from build123d import *

# Parameters (mm, degrees)
F0_R     = 3.175
F0_R_2   = 1.5875
F1_DEPTH = 25.4


with BuildPart() as f1:
    # F0 (on Front) → F1 (new body)
    with BuildSketch(Plane.XZ):
        with BuildLine():
            ThreePointArc((-9.525, 70.523976), (0, 60.998976), (9.525, 70.523976))
            ThreePointArc((9.525, 70.523976), (0, 80.048976), (-9.525, 70.523976))
        make_face()
        with Locations((0, 70.523976)):
            Circle(F0_R, mode=Mode.SUBTRACT)
        with BuildLine():
            Line((15.747457, 21.732266), (9.525, 70.523976))
            ThreePointArc((9.525, 70.523976), (0, 60.998976), (-9.525, 70.523976))
            Line((-9.525, 70.523976), (-15.747457, 21.732266))
            ThreePointArc((-15.747457, 21.732266), (0, 35.598976), (15.747457, 21.732266))
        make_face()
        with Locations((-4.959356, 56.249176)):
            Circle(F0_R_2, mode=Mode.SUBTRACT)
        with BuildLine():
            ThreePointArc((15.875, 19.723976), (15.843082, 20.730144), (15.747457, 21.732266))
            ThreePointArc((15.747457, 21.732266), (0, 35.598976), (-15.747457, 21.732266))
            ThreePointArc((-15.747457, 21.732266), (-15.873668, 19.929643), (-15.794203, 18.124357))
            ThreePointArc((-15.794203, 18.124357), (0, 3.848976), (15.794203, 18.124357))
            ThreePointArc((15.794203, 18.124357), (15.854788, 18.923147), (15.875, 19.723976))
        make_face()
        with Locations((0, 19.723976)):
            Circle(F0_R, mode=Mode.SUBTRACT)
        with BuildLine():
            ThreePointArc((15.794203, 18.124357), (0, 3.848976), (-15.794203, 18.124357))
            Line((-15.794203, 18.124357), (-9.525, -43.776024))
            ThreePointArc((-9.525, -43.776024), (0, -34.251024), (9.525, -43.776024))
            ThreePointArc((9.525, -43.776024), (6.970557, -50.267323), (0.677344, -53.27691))
            Line((0.677344, -53.27691), (44.732405, -51.708498))
            ThreePointArc((44.732405, -51.708498), (36.5125, -43.776024), (44.732405, -35.843549))
            Line((44.732405, -35.843549), (18.934103, -34.9251))
            ThreePointArc((18.934103, -34.9251), (13.224974, -32.205044), (11.307223, -26.178844))
            Line((11.307223, -26.178844), (15.794203, 18.124357))
        make_face()
        with BuildLine():
            ThreePointArc((9.525, -43.776024), (0, -34.251024), (-9.525, -43.776024))
            ThreePointArc((-9.525, -43.776024), (-6.735192, -50.511216), (0, -53.301024))
            Line((0, -53.301024), (0.677344, -53.27691))
            ThreePointArc((0.677344, -53.27691), (6.970557, -50.267323), (9.525, -43.776024))
        make_face()
        with Locations((0, -43.776024)):
            Circle(F0_R, mode=Mode.SUBTRACT)
        with BuildLine():
            Line((0.677344, -53.27691), (0, -53.301024))
            ThreePointArc((0, -53.301024), (0.338886, -53.294993), (0.677344, -53.27691))
        make_face()
        with BuildLine():
            ThreePointArc((52.3875, -43.776024), (50.161633, -38.264113), (44.732405, -35.843549))
            ThreePointArc((44.732405, -35.843549), (36.5125, -43.776024), (44.732405, -51.708498))
            ThreePointArc((44.732405, -51.708498), (50.161633, -49.287934), (52.3875, -43.776024))
        make_face()
        with Locations((44.45, -43.776024)):
            Circle(F0_R, mode=Mode.SUBTRACT)
    extrude(amount=F1_DEPTH)


solid = f1.part
Input: part model. Units: mm. Frame: model coordinates. A direction names the side the tool comes from. Give positions to 0.01 mm unless a question says otherwise; leave off trailing zeros. Write each loop counter-clockwise with the first axis right and the second up, starting at its lowest first coordinate (ties: lowest second). Pieces come first, ordered by that corner, then holes. Notation, with made-up numbers: M -9,-3.5 L 11,-3.5 A17 ccw 11,24.5 Z; hole C 27.25,24.5 d5. An arc over 180 degrees is marked long. Write item = value, one per line. Start each with the question number.
1) Cut plane B-B on y = -21.75. Count the separate pieces of the cut face and the enclosed holes in it, then the cut area to 3 significant figures.
2) Draft query along X for faces 1 (the cylindrical face through (0.209, -12.522, 80.047)), 2 (the cylindrical face through (-0.413, -12.522, -40.628)), 3 (the flat face through (-12.703, -12.522, -12.393)). Return one class per face: +X half, -X half, draft (parallel to the pull), parting line (faces both ways), or undercut.
3) Reachability of faces 4 (the flat face through (3, 0, -1)), 5 (the flat face through (13.52, -12.52, -4.34)) from +Z, -Z, +X, -X, +Y, -Y: full face, straight path, thin tool, end or side. Return the list, or none.
4) Cut plane A-A on x = -5. Return the cut outline in (y, z), then the cut area to 3 significant figures.
5) Material intervals for line 1 along Z through (x, y) = (44.45, -19.5); line 2 along X through (y, z) = (-21.75, -45.5); line 3 along X through (y, z) = (-19.25, 22), sorted ascending. Write a range as [from, to].
6) Cut plane D-D on z = 42. Return the cut outline in (x, y), then the cut area to 3 significant figures.
7) Cut plane C-C on x = 27. Return the cut outline in (y, z).
8) First-contact query: pin 1 Ø10 at (y, z) = (-3, 34) entering from +X; pin 2 Ø1.5 at (y, z) = (-17, 21.5) entering from -X; pin 3 Ø5 at (y, z) = (-22.5, -14.5) entering from -X. Flat tips, straight axial feed; report the tip coordinate or a pass-through.
Solved:
q1.separate_pieces = 1
q1.enclosed_holes = 5
q1.area = 3,790 mm2
q2.face_1 = parting line
q2.face_2 = undercut
q2.face_3 = -X half
q3.face_4 = +Z, -Z, +X, -X, +Y
q3.face_5 = +X, +Y, -Y
q4.outline = M -25.4,-51.88 L 0,-51.88 L 0,54.66 L -25.4,54.66 Z; M -25.4,57.84 L 0,57.84 L 0,78.63 L -25.4,78.63 Z
q4.area = 3,230 mm2
q5.line_1 = [-51.72, -46.95], [-40.6, -35.83]
q5.line_2 = [-9.37, -2.67], [2.67, 41.78], [47.12, 52.2]
q5.line_3 = [-15.71, -2.21], [2.21, 15.71]
q6.outline = M -13.16,-25.4 L 13.16,-25.4 L 13.16,0 L -13.16,0 Z
q6.area = 669 mm2
q7.outline = M -25.4,-52.34 L 0,-52.34 L 0,-35.21 L -25.4,-35.21 Z
q8.pin_1 = 14.82
q8.pin_2 = -15.84
q8.pin_3 = -12.74
